Can you work these out from the drawing? Everything is in mm from the part's minimum corner. Coordinates: 2 decimals unless noted, no trailing zeros. Loops run counter-clockwise (first coordinate to the right, second up) from the corner with the lowest first, then second, coordinate; pieces in that order, holes last. Notation, with made-up numbers: (16, -24.5) - (72, -24.5) arc R19 ccw to (72, 9.5) - close; hole circle Ø10 at (39.25, 34). An arc over 180 degrees is marked (long way). One line per question, with ' | ' between items. Start each with the question number.
1. I'm going to push a flat-ended pin straight in: P1, Ø6.5, axis at x = 15.875, y = 12.7, coming from the -Z side. Where does the tip first touch, or does it pass through?
2. I want a section at A-A, the plane y = 12.7. Write out the boundary of the cut face in (x, z).
3. I want a section at B-B, the plane z = 1.5. Write out the boundary of the cut face in (x, y) (1 decimal), then the cut area to 3 significant figures.
4. I want a section at C-C, the plane x = 16. Write out the boundary of the cut face in (y, z), then the cut area to 3 significant figures.
5. Please list where these lines run through material, in increasing order: L1, parallel to Y at x = 12.5, z = 4 (1 decimal); L2, parallel to X at y = 24.25, z = 4.5 (1 decimal); L3, parallel to Y at x = 18.5, z = 0.75 (1 decimal). Write a range as [from, to].
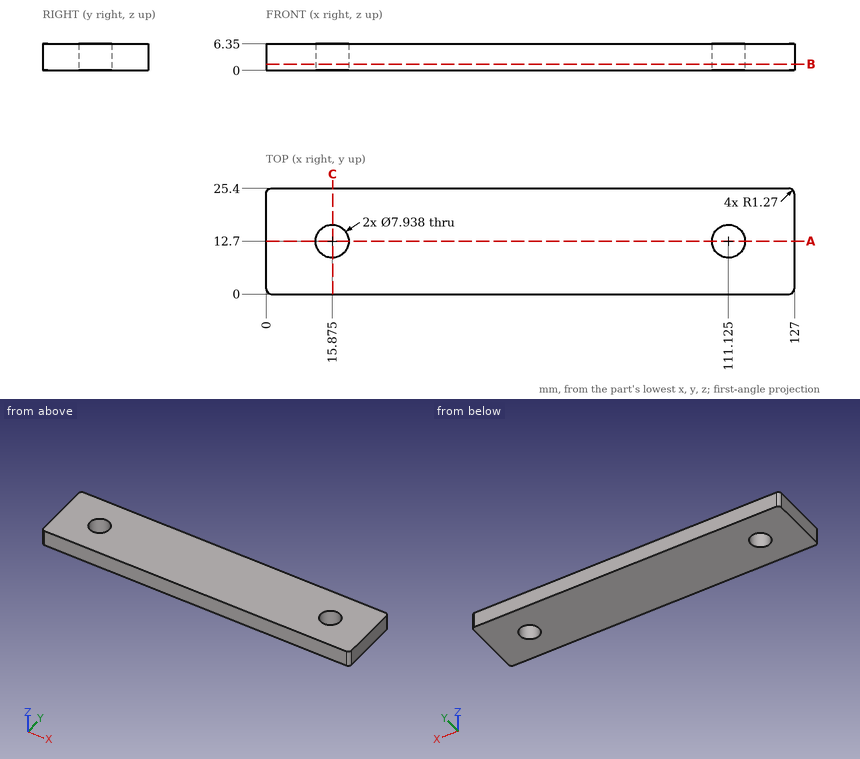
Results are:
1) P1: passes through
2) outline: (0, 0) - (11.91, 0) - (11.91, 6.35) - (0, 6.35) - close; (19.84, 0) - (107.16, 0) - (107.16, 6.35) - (19.84, 6.35) - close; (115.09, 0) - (127, 0) - (127, 6.35) - (115.09, 6.35) - close
3) outline: (0, 1.3) arc R1.3 ccw to (1.3, 0) - (125.7, 0) arc R1.3 ccw to (127, 1.3) - (127, 24.1) arc R1.3 ccw to (125.7, 25.4) - (1.3, 25.4) arc R1.3 ccw to (0, 24.1) - close; hole circle Ø7.9 at (15.9, 12.7); hole circle Ø7.9 at (111.1, 12.7) | area: 3,130 mm2
4) outline: (0, 0) - (8.73, 0) - (8.73, 6.35) - (0, 6.35) - close; (16.67, 0) - (25.4, 0) - (25.4, 6.35) - (16.67, 6.35) - close | area: 111 mm2
5) L1: y = [0, 10.6], [14.8, 25.4] | L2: x = [0, 127] | L3: y = [0, 9.7], [15.7, 25.4]
